CAD build for the part. Positions are in the model's coordinates, mm. A direction names the side the tool comes from. Coordinates: 2 decimals unless noted, no trailing zeros. Loops run counter-clockwise (first coordinate to the right, second up) from the corner with the lowest first, then second, coordinate; pieces in that order, holes last. Notation, with made-up numbers: (12.5, 32.5) -> (58.5, 32.5) arc R23 ccw to (58.5, 50.5) -> close; hole circle Ø2 at (-0.75, -18.5). An arc over 180 degrees is marked (long way). Write each question's results on one line, items separated by ' | '.
from build123d import *

# Parameters (mm, degrees)
F5_R = 6


with BuildPart() as f6:
    # F6: sweep along a path in F0, F4, F2
    with BuildLine(Plane.XY) as f6_path:
        Line((0, 0), (5, 0))
        ThreePointArc((5, 0), (12.0710678119, -2.9289321881), (15, -10))
        Line((15, -10), (15, -18.124))
    with BuildLine(Plane.YZ.offset(15)) as f6_path_2:
        ThreePointArc((-18.124, 0), (-25.1950678119, -2.9289321881), (-28.124, -10))
        Line((-28.124, -10), (-28.124, -20))
    with BuildLine(Plane.XZ.offset(28.124)) as f6_path_3:
        Line((15, -20), (15, -270.5))
        ThreePointArc((15, -270.5), (20.8578643763, -284.6421356237), (35, -290.5))
        Line((35, -290.5), (159.5, -290.5))
    # F5 (on Right) → F6 (sweep)
    with BuildSketch(Plane.YZ):
        Circle(F5_R)
    sweep(path=f6_path.line + f6_path_2.line + f6_path_3.line)


solid = f6.part
1) Slice it at B-B (z = -40). Write the cut outline in (x, y).
Outcome:
outline: circle Ø12 at (15, -28.12)
2) Which spindle directions (+Z, -Z, +X, -X, +Y, -Y) get a long thin tool onto all of the face, cutting with end or side? Do faces 4 (the cylindrical face through (98.12, -29.93, -284.78)), 5 (the flat face through (159.5, -28, -291)), 6 (the cylindrical face through (3, -6, 0)). Say none if no direction does.
Outcome:
face 4: +X | face 5: +Z, -Z, +X, +Y, -Y | face 6: -X
3) Drill centre lines: L1, parallel to Z at x = 47.5, y = -23; L2, parallel to Z at x = 14, y = -28.5; L3, parallel to X at y = -24.5, z = -73.5. Where is each one in solid material? Low to high. Write a range as from..to.
Outcome:
L1: z = -293.62..-287.38 | L2: z = -285.81..2.07 | L3: x = 10.22..19.78
4) Pin check, flat tip, straight feed: pin 1 (8 mm diameter, centred on y = -23, z = -187, fed in from -X). Stop position of the tip, or through.
Outcome:
pin 1: stops at x = 9.11
5) Slice it at A-A (y = -14.5). Write the cut outline in (x, z).
Outcome:
outline: circle Ø12 at (15, 0)
6) Two-plate mould, pull along Y, no slides. Class faces 1 (the cylindrical face through (18.2, -33.2, -142.1)), 2 (the cylindrical face through (20.54, -14.12, -2.3)), 3 (the flat face through (0, 0, 0)): pulls with the +Y half, pulls with the -Y half, needs draft (parallel to the pull), parting line crosses it, or undercut.
Outcome:
face 1: parting line crosses it | face 2: undercut | face 3: needs draft
